For this review, take the finished solid that the model builds, in its own axes (mm). Coordinates: 2 decimals unless noted, no trailing zeros. Write each loop counter-clockwise with the first axis right and the second up, starting at its lowest first coordinate (ties: lowest second). Pieces come first, ordered by that corner, then holes. Notation, with made-up numbers: (-4.75, -12.5) - (18.25, -12.5) arc R16 ccw to (18.25, -4.5) - close; hole circle Ø11 at (77, 22.5). An arc over 180 degrees is marked (long way). Write each question's results on one line, items separated by ' | '.
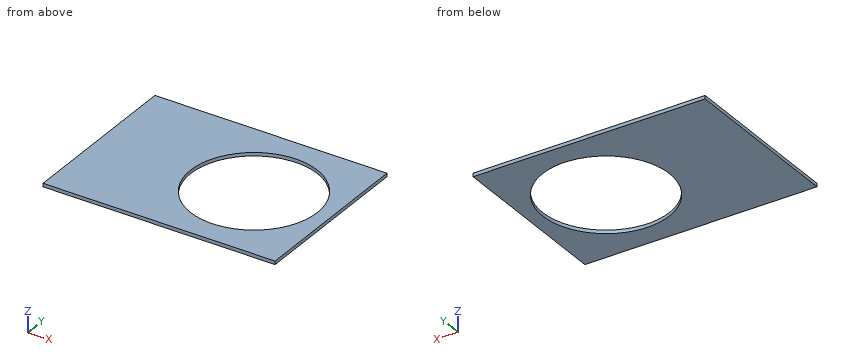
from build123d import *

# Parameters (mm, degrees)
BOSS_EXTRUDE1_DEPTH = 0.254
SKETCH2_R           = 4.699
CUT_EXTRUDE1_DEPTH  = 1.254
SKETCH3_W           = 2.54
SKETCH3_H           = 0.635
CUT_EXTRUDE2_DEPTH  = 1.254
SKETCH5_OUTSIDE_W   = 121.447
SKETCH5_OUTSIDE_H   = 109.618
SKETCH5_OUTSIDE_W_2 = 17.2085
SKETCH5_OUTSIDE_H_2 = 15.24
CUT_EXTRUDE5_DEPTH  = 1.254


with BuildPart() as part:
    # Sketch1 → Boss-Extrude1 (new body)
    with BuildSketch(Plane.XY):
        with BuildLine():
            Line((67.21146711, 76.191723231), (8.696654013, 17.676910134))
            Line((8.696654013, 17.676910134), (7.228954972, 14.133571205))
            ThreePointArc((7.228954972, 14.133571205), (14.666587579, 6.075099489), (15.105587123, -4.88230096))
            Line((15.105587123, -4.88230096), (18.648926052, -6.35))
            Line((18.648926052, -6.35), (101.401368334, -6.35))
            ThreePointArc((101.401368334, -6.35), (93.866160503, 38.880636728), (67.21146711, 76.191723231))
        make_face()
        with BuildLine():
            Line((88.672924278, 6.35), (27.86051193, 6.35))
            ThreePointArc((27.86051193, 6.35), (26.399857642, 10.93517908), (24.190484974, 15.210228852))
            Line((24.190484974, 15.210228852), (67.191354125, 58.211098004))
            ThreePointArc((67.191354125, 58.211098004), (82.13289044, 34.020557137), (88.672924278, 6.35))
        make_face(mode=Mode.SUBTRACT)
    extrude(amount=BOSS_EXTRUDE1_DEPTH)

    # Sketch2 → Cut-Extrude1 (cut, through all)
    with BuildSketch(Plane.XY.offset(0.254)):
        with Locations((22.225, 0)):
            Circle(SKETCH2_R)
        with Locations((36.195, 0)):
            Circle(SKETCH2_R)
        with Locations((61.722, 0)):
            Circle(SKETCH2_R)
        with Locations((75.692, 0)):
            Circle(SKETCH2_R)
        with Locations((95.25, 0)):
            Circle(SKETCH2_R)
        with Locations((15.715448212, 15.715448212)):
            Circle(SKETCH2_R)
        with Locations((25.593729945, 25.593729945)):
            Circle(SKETCH2_R)
        with Locations((43.644044748, 43.644044748)):
            Circle(SKETCH2_R)
        with Locations((53.522326482, 53.522326482)):
            Circle(SKETCH2_R)
        with Locations((92.004434954, 24.652514046)):
            Circle(SKETCH2_R)
        with Locations((82.48891971, 47.625)):
            Circle(SKETCH2_R)
        with Locations((67.351920908, 67.351920908)):
            Circle(SKETCH2_R)
    extrude(amount=-CUT_EXTRUDE1_DEPTH, mode=Mode.SUBTRACT)

    # Sketch3 → Cut-Extrude2 (cut, through all)
    with BuildSketch(Plane.XY.offset(0.254)):
        Polygon((15.266435406, 24.246691527), (17.06248663, 26.042742751), (17.511499436, 25.593729945), (15.715448212, 23.797678721), align=None)
        Polygon((44.991083167, 53.971339288), (43.195031942, 52.175288063), (43.644044748, 51.726275257), (45.440095973, 53.522326482), align=None)
        with Locations((29.21, -6.0325)):
            Rectangle(SKETCH3_W, SKETCH3_H)
        with Locations((68.707, -6.0325)):
            Rectangle(SKETCH3_W, SKETCH3_H)
        Polygon((29.230733674, 38.210989795), (31.026784898, 40.007041019), (31.475797704, 39.558028213), (29.67974648, 37.761976989), align=None)
        Polygon((56.845021246, 65.825277367), (55.048970022, 64.029226143), (55.497982828, 63.580213337), (57.294034052, 65.376264561), align=None)
        with Locations((48.9585, -6.0325)):
            Rectangle(SKETCH3_W, SKETCH3_H)
        with Locations((85.471, -6.0325)):
            Rectangle(SKETCH3_W, SKETCH3_H)
        Polygon((99.935462164, 14.437711971), (100.266998693, 11.919442024), (101.526133667, 12.085210288), (101.194597138, 14.603480236), align=None)
        Polygon((93.765504959, 37.464305742), (94.938831965, 37.950313702), (93.966816047, 40.296967714), (92.793489041, 39.810959755), align=None)
        Polygon((79.327792988, 62.471156422), (80.874047017, 60.456038938), (81.88160576, 61.229165953), (80.33535173, 63.244283437), align=None)
        Polygon((13.593916116, 7.005422516), (14.565932035, 4.658768503), (15.739259041, 5.144776462), (14.767243123, 7.491430475), align=None)
    extrude(amount=-CUT_EXTRUDE2_DEPTH, mode=Mode.SUBTRACT)

    # Sketch5 outside → Cut-Extrude5 (cut, through all)
    with BuildSketch(Plane.XY.offset(0.254)):
        with Locations((54.4145, 34.921)):
            Rectangle(SKETCH5_OUTSIDE_W, SKETCH5_OUTSIDE_H)
        with Locations((58.83275, 0)):
            Rectangle(SKETCH5_OUTSIDE_W_2, SKETCH5_OUTSIDE_H_2, mode=Mode.SUBTRACT)
    extrude(amount=-CUT_EXTRUDE5_DEPTH, mode=Mode.SUBTRACT)


solid = part.part
Q1. Take a section at A-A on y = 0. State the section outline as (x, z) points.
Results found:
outline: (50.23, 0) - (57.02, 0) - (57.02, 0.25) - (50.23, 0.25) - close; (66.42, 0) - (67.44, 0) - (67.44, 0.25) - (66.42, 0.25) - close
Q2. Wall thickness on line 1 along X through (y, z) = (1.5, 0.15); line 2 along X through (y, z) = (-0.5, 0.1); line 3 along Y through (x, z) = (66, 0.2): over which ranges is each line inside the solid? List them lowest first. Write a range as from..to.
Results found:
line 1: 50.23..57.27, 66.18..67.44 | line 2: 50.23..57.05, 66.39..67.44 | line 3: -6.35..-1.94, 1.94..6.35
Q3. Take a section at C-C on z = 0.2. State the section outline as (x, y) points.
Results found:
outline: (50.23, -6.35) - (67.44, -6.35) - (67.44, 6.35) - (50.23, 6.35) - close; hole circle Ø9.4 at (61.72, 0)
Q4. Take a section at B-B on x = 64.25. State the section outline as (y, z) points.
Results found:
outline: (-6.35, 0) - (-3.96, 0) - (-3.96, 0.25) - (-6.35, 0.25) - close; (3.96, 0) - (6.35, 0) - (6.35, 0.25) - (3.96, 0.25) - close
